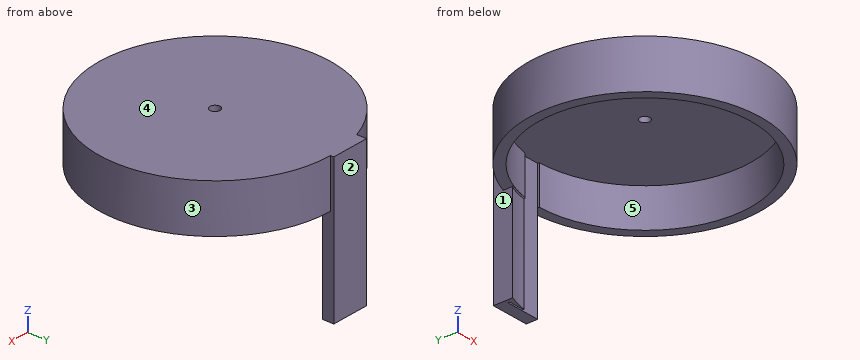
Autodesk Inventor part; units mm, degrees
ref_plane "YZ Plane" through (0, 0, 0) normal (1, 0, 0) x (0, 1, 0)
ref_plane "XZ Plane" through (0, 0, 0) normal (0, 1, 0) x (-1, 0, 0)
ref_plane "XY Plane" through (0, 0, 0) normal (0, 0, 1) x (1, 0, 0)
sketch "Sketch1" plane through (0, 0, 0) normal (0, 0, 1) x (1, 0, 0)
  circle A0 centre (0, 0) radius 60
  circle A1 centre (0, 0) radius 2.65
  dimension "d0" = 120
  dimension "d1" = 5.3
extrude "Extrusion1" add sketch "Sketch1" along normal blind 5
sketch "Sketch4" plane through (0, 0, 0) normal (0, 0, -1) x (-1, 0, 0)
  circle A0 centre (0, 0) radius 2.65
  circle A1 centre (0, 0) radius 54.85
  circle A2 centre (0, 0) radius 60
  dimension "d13" = 109.7
  dimension "d14" = 120
extrude "Extrusion4" add sketch "Sketch4" along normal blind 20 contours A2
sketch "Sketch7" plane through (0, 0, -20) normal (0, 0, -1) x (-1, 0, 0)
  circle A0 centre (0, 0) radius 54.85
  line L0 (0, 54.85) -> (30.5637, 54.85)
  line L1 (30.5637, 54.85) -> (30.5637, 55.75)
  line L2 (30.5637, 55.75) -> (0, 55.75)
  line L3 (0, 55.75) -> (0, 54.85)
  line L4 (18, 55.75) -> (18, 54.85)
  line L5 (4.9967, 54.85) -> (4.9967, 54.185)
  line L6 (4.9967, 54.185) -> (0, 54.85)
  dimension "d25" = 0.9
extrude "Extrusion7" cut sketch "Sketch7" against normal blind 20 contours L0 L5 A0 | L3 L2 L4 L0 | A0 L5 L6 picked at (2.2214, 54.6199)
sketch "Sketch8" plane through (0, 0, -20) normal (0, 0, -1) x (-1, 0, 0)
  arc A0 (0, 54.85) -> (4.9967, 54.6219) centre (0, 0) ccw
  line L0 (19.9252, 51.1029) -> (19.9252, 61.7106)
  line L1 (19.9252, 61.7106) -> (0, 61.7106)
  line L2 (0, 55.75) -> (18, 55.75)
  line L3 (0, 61.7106) -> (0, 55.75)
  line L4 (0, 55.75) -> (18, 55.75)
  line L5 (18, 55.75) -> (18, 54.85)
  line L6 (18, 55.75) -> (18, 54.85)
  line L7 (18, 54.85) -> (4.9967, 54.85)
  line L8 (4.9967, 54.85) -> (4.9967, 54.6219)
  line L9 (4.9967, 54.85) -> (4.9967, 54.6219)
  line L10 (18, 54.85) -> (4.9967, 54.85)
  line L11 (7.5379, 54.85) -> (7.5379, 54.3296)
  arc A1 (19.9685, 51.6391) -> (7.5379, 54.85) centre (0, 0) ccw
  line L12 (9.6264, 54.85) -> (9.6264, 54.5222)
  point P0 (19.9252, 51.6559)
extrude "Extrusion8" add sketch "Sketch8" along normal blind 50 and the other way blind 25 contours A1 L12 L7 L5 L2 L3 L1 L0
chamfer "Chamfer1" distance 0.5 angle 45 1 edges at (-14.8452, 53.3382, -20)
sketch "Sketch9" plane through (0, 0, -20) normal (0, 0, -1) x (-1, 0, 0)
  line L0 (9.6264, 54.0144) -> (9.6264, 54.85)
  line L1 (9.6264, 54.85) -> (4.9967, 54.85)
  line L2 (9.6264, 54.85) -> (4.9967, 54.85)
  line L3 (4.9967, 54.85) -> (4.9967, 54.6219)
  line L4 (4.9967, 54.85) -> (4.9967, 54.6219)
  line L5 (4.9967, 54.6219) -> (4.9967, 54.2488)
  line L6 (4.9967, 54.2488) -> (9.6264, 53.9987)
  arc A0 (0, 54.85) -> (4.9967, 54.6219) centre (0, 0) ccw
  line L7 (9.6264, 54.85) -> (9.6264, 53.9987)
extrude "Extrusion9" cut sketch "Sketch9" against normal blind 20
properties part number "Disc"
Verification items for the finished model (mm, model axes). Face numbers are marked on the shaded views. A direction names the side the tool comes from. Coordinates: 2 decimals unless noted, no trailing zeros. Loops run counter-clockwise (first coordinate to the right, second up) from the corner with the lowest first, then second, coordinate; pieces in that order, holes last. Notation, with made-up numbers: (-5, -32.75) - (4, -32.75) arc R29 cw to (4, -9.75) - close; hole circle Ø7 at (3, 14). An arc over 180 degrees is marked (long way). Answer as a JSON object with one key per item and string values.
(1) Cross-section at B-B, the plane z = -38. Record the boundary of the cut face in (x, y).
Response:
{"outline": "(-19.93, 51.66) arc R55.37 cw to (-9.63, 54.52) - (-9.63, 54.85) - (-18, 54.85) - (-18, 55.75) - (0, 55.75) - (0, 61.71) - (-19.93, 61.71) - close"}
(2) Cross-section at C-C, the plane x = 15. Record the boundary of the cut face in (y, z), then the cut area to 3 significant figures.
Response:
{"outline": "(-58.09, -20) - (-52.76, -20) - (-52.76, 0) - (52.76, 0) - (52.76, -20) - (58.09, -20) - (58.09, 5) - (-58.09, 5) - close", "area": "794 mm²"}
(3) Cross-section at A-A, the plane y = 0. Record the boundary of the cut face in (x, z), then the cut area to 4 significant figures.
Response:
{"outline": "(-60, -20) - (-54.85, -20) - (-54.85, 0) - (-2.65, 0) - (-2.65, 5) - (-60, 5) - close; (2.65, 0) - (54.85, 0) - (54.85, -20) - (60, -20) - (60, 5) - (2.65, 5) - close", "area": "779.5 mm²"}
(4) Mould release check, pull along Y, two halves, no side actions. Record for the marked faces 3, 4 and 5: pulls with the +Y half, pulls with the -Y half, needs draft (parallel to the pull), parting line crosses it, or undercut.
Response:
{"face 3": "parting line crosses it", "face 4": "needs draft", "face 5": "undercut"}
(5) Scan lines: line 1 along X through (y, z) = (0, -4.25); line 2 along Y through (x, z) = (-16.5, -12.5); line 3 along Z through (x, y) = (-52.5, -25.5). Record each from-to range of solid material in increasing order.
Response:
{"line 1": "x = -60 to -54.85, 54.85 to 60", "line 2": "y = -57.69 to -52.31, 52.31 to 54.85, 55.75 to 61.71", "line 3": "z = -20 to 5"}
(6) Go/stop test with flat-tipped pins: pin 1 Ø1.5 at (x, z) = (37, -11) entering from -Y; pin 2 Ø4 at (y, z) = (-6.5, -6.5) entering from -X; pin 3 Ø4 at (x, z) = (39.5, -12.5) entering from -Y; pin 4 Ø6 at (x, y) = (0, 0) entering from +Z. Record where each tip stops, or that it passes through.
Response:
{"pin 1": "stops at y = -47.81", "pin 2": "stops at x = -59.83", "pin 3": "stops at y = -46.84", "pin 4": "stops at z = 5"}
(7) Cross-section at D-D, the plane z = -16. Record the boundary of the cut face in (x, y), then the cut area to 3 significant figures.
Response:
{"outline": "(-19.93, 56.59) arc R60 ccw (long way) to (0, 60) - (0, 61.71) - (-19.93, 61.71) - close; hole (-18, 54.85) - (-9.63, 54.85) - (-9.63, 54) arc R54.85 ccw (long way) to (0, 54.85) - (0, 55.75) - (-18, 55.75) - close", "area": "1,900 mm²"}
(8) Access from +Z, -Z, +X, -X, +Y, -Y to the whole of each face (thin tool, end or side, straight path). Record for the marked faces 1 and 2.
Response:
{"face 1": "-Z, -X, +Y", "face 2": "+Z, -Z, +X, -X, +Y"}
